Input: part model. Units: mm. Frame: model coordinates. Coordinates: 2 decimals unless noted, no trailing zeros. Loops run counter-clockwise (first coordinate to the right, second up) from the corner with the lowest first, then second, coordinate; pieces in that order, holes last.
Item 1: Section B-B on x = 39.5. Return loops of the section in (y, z), and give its area (3 significant figures).
Item 2: Ray query, line 1 along Z through (x, y) = (58.5, -1500); line 2 along X through (y, z) = (-1466.5, -0.75); line 3 along X through (y, z) = (-1549.5, 0). Return the intervals inside material, ascending.
Item 3: Contact query for flat-ended pins moving along their axis: P1, Ø4, axis at x = 93.5, z = 0, coming from the +Y side; P2, Ø3, axis at x = 36, z = -2, coming from the +Y side; P3, Ø4, axis at x = 72.5, z = -6, coming from the -Y side. Output: stop coordinate, or through.
Item 4: Section C-C on y = -849.5. Return loops of the section in (x, z), and give its area (3 significant figures).
Item 5: Section A-A on z = 0. Return loops of the section in (x, y), and give its area (3 significant figures).
```python
from build123d import *

# Parameters (mm, degrees)
F0_R     = 7.5
F0_R_2   = 5.5
F3_DEPTH = 17.2466


with BuildPart() as f2:
    # F2: sweep along a path in F1
    with BuildLine(Plane.XY) as f2_path:
        Line((0, 0), (0, -1480))
        ThreePointArc((0, -1480), (5.8578643763, -1494.1421356237), (20, -1500))
        Line((20, -1500), (80, -1500))
        ThreePointArc((80, -1500), (94.1421356237, -1505.8578643763), (100, -1520))
        Line((100, -1520), (100, -1600))
    # F0 (on Front) → F2 (sweep)
    with BuildSketch(Plane.XZ):
        Circle(F0_R)
        Circle(F0_R_2, mode=Mode.SUBTRACT)
    sweep(path=f2_path.line)

    # F3 (add): a face of the model
    f3_faces = [f2.faces().sort_by_distance(p)[0] for p in [
        (-7.2878679656, 0, 0),
    ]]
    extrude(f3_faces, amount=F3_DEPTH)


solid = f2.part
```
Results found:
1. outline: circle Ø15 at (-1500, 0); hole circle Ø11 at (-1500, 0)
1. area: 81.7 mm2
2. line 1: z = -7.5 to -5.5, 5.5 to 7.5
2. line 2: x = -7.46 to -5.45, 5.45 to 7.46
2. line 3: x = 92.5 to 94.5, 105.5 to 107.5
3. P1: stops at y = -1495.02
3. P2: stops at y = -1492.52
3. P3: stops at y = -1506.34
4. outline: circle Ø15 at (0, 0); hole circle Ø11 at (0, 0)
4. area: 81.7 mm2
5. outline: (-7.5, -1480) arc R27.5 ccw to (20, -1507.5) - (80, -1507.5) arc R12.5 cw to (92.5, -1520) - (92.5, -1600) - (94.5, -1600) - (94.5, -1520) arc R14.5 ccw to (80, -1505.5) - (20, -1505.5) arc R25.5 cw to (-5.5, -1480) - (-5.5, 17.25) - (-7.5, 17.25) - close; (5.5, -1480) arc R14.5 ccw to (20, -1494.5) - (80, -1494.5) arc R25.5 cw to (105.5, -1520) - (105.5, -1600) - (107.5, -1600) - (107.5, -1520) arc R27.5 ccw to (80, -1492.5) - (20, -1492.5) arc R12.5 cw to (7.5, -1480) - (7.5, 17.25) - (5.5, 17.25) - close
5. area: 6,800 mm2
